from build123d import *

# Parameters (mm, degrees)
SKETCH1_W           = 170
SKETCH1_H           = 160
BOSS_EXTRUDE2_DEPTH = 50
CUT_EXTRUDE2_REACH  = 189.949
SKETCH3_W           = 160
SKETCH3_H           = 40
CUT_EXTRUDE3_REACH  = 128.984
SKETCH4_W           = 150
SKETCH4_H           = 160


with BuildPart() as part:
    # Sketch1 → Boss-Extrude2 (new body)
    with BuildSketch(Plane(origin=(0, 0, 0), x_dir=(1, 0, 0), z_dir=(0, 1, 0))):
        Rectangle(SKETCH1_W, SKETCH1_H)
    extrude(amount=BOSS_EXTRUDE2_DEPTH)

    # Sketch3 → Cut-Extrude2 (cut, up to next)
    with BuildSketch(Plane.XY.offset(80), mode=Mode.PRIVATE) as cut_extrude2_sk1:
        with Locations((0, 25)):
            Rectangle(SKETCH3_W, SKETCH3_H)
    cut_extrude2_tool1 = extrude(cut_extrude2_sk1.sketch, amount=-CUT_EXTRUDE2_REACH, mode=Mode.PRIVATE) & part.part
    add(cut_extrude2_tool1.solids().sort_by_distance((0, 25, 80))[0], mode=Mode.SUBTRACT)

    # Sketch4 → Cut-Extrude3 (cut, up to next)
    with BuildSketch(Plane(origin=(0, 50, 0), x_dir=(1, 0, 0), z_dir=(0, 1, 0)), mode=Mode.PRIVATE) as cut_extrude3_sk1:
        Rectangle(SKETCH4_W, SKETCH4_H)
    cut_extrude3_tool1 = extrude(cut_extrude3_sk1.sketch, amount=-CUT_EXTRUDE3_REACH, mode=Mode.PRIVATE) & part.part
    add(cut_extrude3_tool1.solids().sort_by_distance((0, 50, 0))[0], mode=Mode.SUBTRACT)


solid = part.part
Geometry check sheet. Reference: the model listing, model coordinates, mm. A direction names the side the tool comes from. Round coordinates to 2 decimals unless told otherwise and drop trailing zeros. Write each loop counter-clockwise with the first axis right and the second up, starting at its lowest first coordinate (ties: lowest second). Pieces come first, ordered by that corner, then holes. Notation, with made-up numbers: (42, -30.5) - (79, -30.5) arc R12 ccw to (79, -19.5) - close; hole circle Ø5 at (-12.5, -10.75). An arc over 180 degrees is marked (long way). One line per item, written item: value.
1. Mould release check, pull along Y, two halves, no side actions. Record for faces 1 (the face through (-1, 0, -1)), 2 (the face through (-78, 45, 1)), 3 (the face through (-75, 48, 1)): released by +Y, released by -Y, zero draft, split by the parting line, or undercut.
The answers:
face 1: released by -Y
face 2: undercut
face 3: zero draft
2. Set-up check for faces 4 (the face through (75, 48, 1)), 5 (the face through (-0.4, 4.5, 80)), 6 (the face through (77, 45, 1)): record each of +Z, -Z, +X, -X, +Y, -Y from which the full face is reachable in a straight line by a thin tool's end or side.
The answers:
face 4: +Z, -Z, +Y
face 5: +Z, +X, -X, +Y, -Y
face 6: +Z, -Z
3. Depth check by flat-ended pin: pin 1 Ø10 at (x, z) = (-68, 36) entering from +Y. Enter the tip coordinate at first touch or a pass-through.
The answers:
pin 1: stops at y = 5
4. Cross-section at A-A on y = 10. Record the boundary of the cut face in (x, z), and give its area (3 significant figures).
The answers:
outline: (-85, -80) - (-80, -80) - (-80, 80) - (-85, 80) - close; (80, -80) - (85, -80) - (85, 80) - (80, 80) - close
area: 1,600 mm^2
5. Scan lines: L1, parallel to X at y = 32, z = -8; L2, parallel to X at y = 47.5, z = 53; L3, parallel to Y at x = 30, z = 23. Record each from-to range of solid material in increasing order.
The answers:
L1: x = -85 to -80, 80 to 85
L2: x = -85 to -75, 75 to 85
L3: y = 0 to 5
6. Cross-section at C-C on x = -35. Record the boundary of the cut face in (y, z), and give its area (3 significant figures).
The answers:
outline: (0, -80) - (5, -80) - (5, 80) - (0, 80) - close
area: 800 mm^2
7. Cross-section at B-B on z = -3. Record the boundary of the cut face in (x, y).
The answers:
outline: (-85, 0) - (85, 0) - (85, 50) - (75, 50) - (75, 45) - (80, 45) - (80, 5) - (-80, 5) - (-80, 45) - (-75, 45) - (-75, 50) - (-85, 50) - close
